Geometry: see drawing. Coordinates: mm, zero at the bounding-box minimum. Coordinates: 2 decimals unless noted, no trailing zeros. Loops run counter-clockwise (first coordinate to the right, second up) from the corner with the lowest first, then second, coordinate; pieces in that order, holes last.
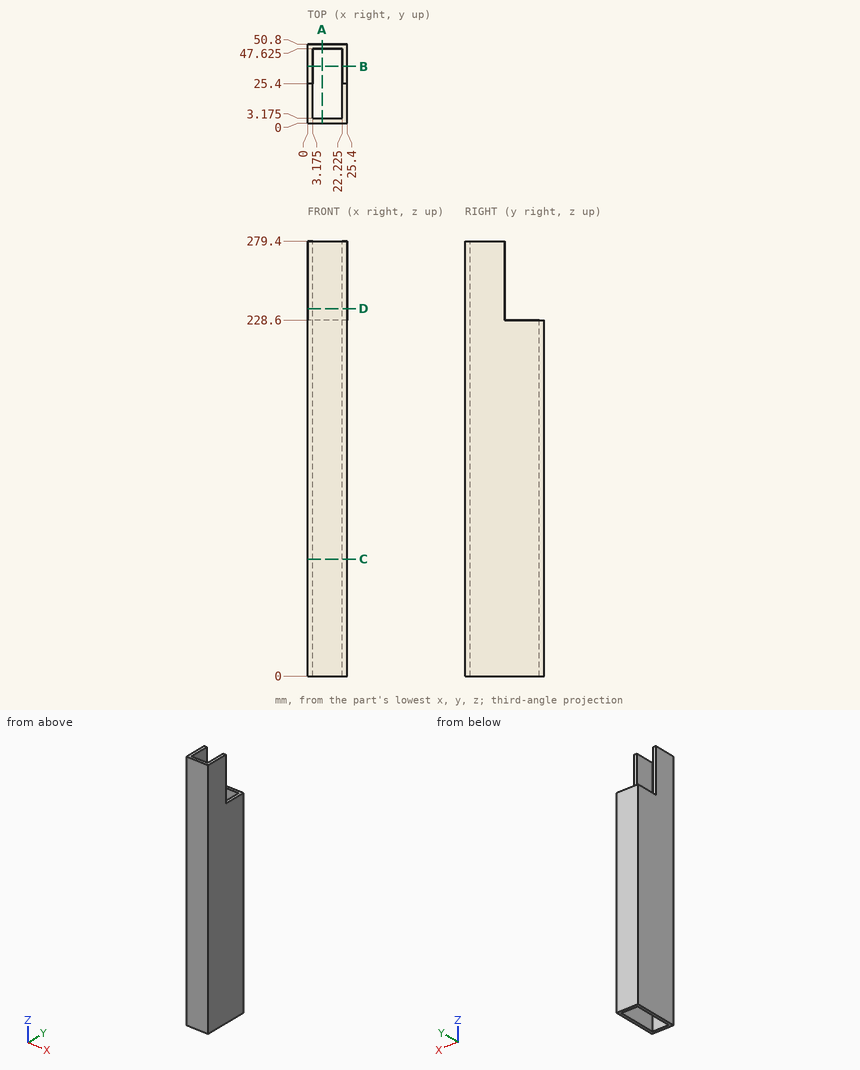
Item 1: Section query C-C (z = 75). Output: boundary loops of the cut face in (x, y) (3 decimals).
Result:
outline: (0, 0) - (25.4, 0) - (25.4, 50.8) - (0, 50.8) - close; hole (3.175, 3.175) - (22.225, 3.175) - (22.225, 47.625) - (3.175, 47.625) - close
Item 2: Section query D-D (z = 236). Output: boundary loops of the cut face in (x, y) (3 decimals), then the cut area to 3 significant figures.
Result:
outline: (0, 0) - (25.4, 0) - (25.4, 25.4) - (22.225, 25.4) - (22.225, 3.175) - (3.175, 3.175) - (3.175, 25.4) - (0, 25.4) - close
area: 222 mm2
Item 3: Contact query for flat-ended pins moving along their axis: P1, Ø8, axis at x = 18, y = 13, coming from the +Z side; P2, Ø12, axis at x = 11, y = 42.5, coming from the +Z side; P3, Ø6, axis at x = 7.5, z = 210, coming from the -Y side; P4, Ø2.5, axis at x = 24.5, z = 246, coming from the +Y side. Output: stop coordinate, or through.
Result:
P1: passes through
P2: stops at z = 228.6
P3: stops at y = 0
P4: stops at y = 25.4
Item 4: Section query A-A (x = 9.25). Output: boundary loops of the cut face in (y, z) (3 decimals).
Result:
outline: (0, 0) - (3.175, 0) - (3.175, 279.4) - (0, 279.4) - close; (47.625, 0) - (50.8, 0) - (50.8, 228.6) - (47.625, 228.6) - close
Item 5: Section query B-B (y = 36.5). Output: boundary loops of the cut face in (x, z) (3 decimals).
Result:
outline: (0, 0) - (3.175, 0) - (3.175, 228.6) - (0, 228.6) - close; (22.225, 0) - (25.4, 0) - (25.4, 228.6) - (22.225, 228.6) - close
Item 6: Line query: L1, parallel to X at y = 15.5, z = 148 (3 decimals); L2, parallel to Y at x = 3.5, z = 122 (3 decimals); L3, parallel to Y at x = 23, z = 238. Output: solid intervals per line, ascending.
Result:
L1: x = 0 to 3.175, 22.225 to 25.4
L2: y = 0 to 3.175, 47.625 to 50.8
L3: y = 0 to 25.4
